Autodesk Inventor part; units mm, degrees
ref_plane "YZ Plane" through (0, 0, 0) normal (1, 0, 0) x (0, 1, 0)
ref_plane "XZ Plane" through (0, 0, 0) normal (0, 1, 0) x (-1, 0, 0)
ref_plane "XY Plane" through (0, 0, 0) normal (0, 0, 1) x (1, 0, 0)
sketch "Sketch1" plane through (0, 0, 0) normal (0, 1, 0) x (-1, 0, 0)
  line L0 (0, 0) -> (0, -54.7595)
  line L1 (0, -54.7595) -> (17.2816, -61.6681)
  line L2 (0, -54.7595) -> (18.6114, -54.7595) construction
  line L3 (0, -54.7595) -> (28.8848, -66.3067)
  line L4 (28.8848, -66.3067) -> (28.8848, -54.7595)
  line L5 (28.8848, -54.7595) -> (28.8848, 0)
  line L6 (28.8848, 0) -> (28.8848, 11.5473)
  line L7 (28.8848, 11.5473) -> (0, 0)
  line L8 (0, -50.5358) -> (-4, -50.5358)
  line L9 (3.9418, -56.3353) -> (2.457, -60.0495)
  line L10 (2.457, -60.0495) -> (-4, -57.4682)
  line L11 (-4, -57.4682) -> (-4, -50.5358)
  line L12 (28.8848, -66.3067) -> (27.4, -70.0209)
  line L13 (27.4, -70.0209) -> (2.457, -60.0495)
  line L14 (0, -3.5872) -> (-4, -3.5872)
  line L15 (-4, -3.5872) -> (-4, -50.5358)
  line L16 (2.457, 0.9822) -> (0.9721, 4.6964)
  line L17 (0.9721, 4.6964) -> (-4, 2.7087)
  line L18 (-4, 2.7087) -> (-4, -3.5872)
  line L19 (23.3647, 9.3405) -> (21.8799, 13.0547)
  line L20 (21.8799, 13.0547) -> (0.9721, 4.6964)
  line L21 (28.8848, 11.5473) -> (27.4, 15.2615)
  line L22 (27.4, 15.2615) -> (21.8799, 13.0547)
  dimension "d0" = 54.7595
  dimension "d1" = 21.79
  dimension "d2" = 31.1075
  dimension "d3" = 11.5473
  dimension "d4" = 11.5473
  dimension "d5" = 4
  dimension "d6" = 4
  dimension "d7" = 4
extrude "Extrusion1" add sketch "Sketch1" along normal blind 40 contours L0 L14 L18 L17 L16 L7 | L0 L8 L15 L14 | L16 L20 L19 L7 | L0 L1 L9 L10 L11 L8 | L19 L22 L21 L7 | L1 L3 L12 L13 L9
sketch "Sketch2" plane through (0, 0, 0) normal (0, -1, 0) x (1, 0, 0)
  line L0 (0, -54.7595) -> (0, 0)
  line L1 (0, -27.3797) -> (8, -27.3797)
  circle A0 centre (8, -27.3797) radius 1.75
  circle A1 centre (8, -27.3797) radius 3.5
  line L2 (4, 2.7087) -> (4, -57.4682)
  line L3 (4, -27.3797) -> (4, -30.8797)
  line L4 (4, -30.8797) -> (8, -30.8797)
  line L5 (4, -27.3797) -> (4, -23.8797)
  line L6 (4, -23.8797) -> (8, -23.8797)
  line L7 (-27.4, -70.0209) -> (-28.8848, -66.3067)
  line L8 (-28.8848, -66.3067) -> (-27.0288, -70.9495)
  line L9 (-27.0288, -70.9495) -> (-28.8848, -66.3067)
  line L10 (-28.8848, -66.3067) -> (-24.2421, -64.4507)
  line L11 (-24.2421, -64.4507) -> (-21.2724, -71.8791)
  circle A2 centre (-21.2724, -71.8791) radius 1.75
  circle A3 centre (-21.2724, -71.8791) radius 3.5
  line L12 (4, -57.4682) -> (-27.4, -70.0209)
  line L13 (-22.7573, -68.1649) -> (-26.0072, -69.4641)
  line L14 (-26.0072, -69.4641) -> (-24.5224, -73.1783)
  line L15 (-22.7573, -68.1649) -> (-19.5073, -66.8657)
  line L16 (-19.5073, -66.8657) -> (-18.0225, -70.5799)
  line L17 (-28.8848, 11.5473) -> (-24.2421, 9.6912)
  line L18 (0, 0) -> (-28.8848, 11.5473)
  line L19 (-24.2421, 9.6912) -> (-21.2724, 17.1196)
  circle A4 centre (-21.2724, 17.1196) radius 1.75
  circle A5 centre (-21.2724, 17.1196) radius 3.5
  line L20 (-27.4, 15.2615) -> (4, 2.7087)
  line L21 (-22.7573, 13.4054) -> (-26.0072, 14.7047)
  line L22 (-26.0072, 14.7047) -> (-24.5224, 18.4189)
  line L23 (-22.7573, 13.4054) -> (-19.5073, 12.1062)
  line L24 (-19.5073, 12.1062) -> (-18.0225, 15.8204)
  dimension "d10" = 8
  dimension "d11" = 3.5
  dimension "d12" = 7
  dimension "d13" = 5
  dimension "d14" = 5
  dimension "d15" = 8
  dimension "d16" = 3.5
  dimension "d17" = 7
  dimension "d18" = 3.5
  dimension "d19" = 3.5
  dimension "d20" = 5
  dimension "d21" = 3.5
  dimension "d22" = 7
  dimension "d23" = 3.5
extrude "Extrusion2" add sketch "Sketch2" against normal blind 3 contours L16 A3 L11 L12 | L2 L6 A1 L1 | L1 A1 L4 L2 | A1 | L20 L22 A5 L19 | L19 A5 L24 L20 | A5 | L11 A3 L14 L12 | A3
sketch "Sketch3" plane through (0, 40, 0) normal (0, 1, 0) x (1, 0, 0)
  line L0 (4, 23.8797) -> (4, 30.8797)
  line L1 (4, 27.3797) -> (4, 30.8797)
  line L2 (8, 30.8797) -> (4, 30.8797)
  line L3 (4, 30.8797) -> (8, 30.8797)
  line L4 (4, 27.3797) -> (4, 23.8797)
  line L5 (4, 23.8797) -> (8, 23.8797)
  line L6 (4, 23.8797) -> (8, 23.8797)
  circle A0 centre (8, 27.3797) radius 1.75
  circle A1 centre (8, 27.3797) radius 1.75
  circle A2 centre (8, 27.3797) radius 3.5
  point P0 (0, 0)
extrude "Extrusion3" add sketch "Sketch3" against normal blind 3 contours A2
sketch "Sketch4" plane through (0, 40, 0) normal (0, 1, 0) x (1, 0, 0)
  line L0 (4, 23.8797) -> (4, 30.8797)
  line L1 (4, 23.8797) -> (8, 23.8797)
  circle A0 centre (8, 27.3797) radius 3.5
  line L2 (8, 30.8797) -> (4, 30.8797)
  line L3 (4, 30.8797) -> (8, 30.8797)
  point P0 (0, 0)
extrude "Extrusion4" add sketch "Sketch4" against normal blind 3 contours L0 L2 A0 L1
sketch "Sketch5" plane through (0, 40, 0) normal (0, 1, 0) x (1, 0, 0)
  point P0 (0, 0)
fillet "Fillet1" radius 20 4 edges at (0, 20, 0) (0, 20, -54.7595) (4, 20, 2.7087) (4, 20, -57.4682)
properties part number "Capture Zone4"
Build history of the part. All positions in model axes, mm. A direction names the side the tool comes from. Give positions to 0.01 mm unless a question says otherwise; leave off trailing zeros. Loops run counter-clockwise (first coordinate to the right, second up) from the corner with the lowest first, then second, coordinate; pieces in that order, holes last. Notation, with made-up numbers: (77.25, 20.5) - (108.25, 20.5) arc R11 cw to (108.25, 25.5) - close; hole circle Ø9 at (-15.5, 27.5). An arc over 180 degrees is marked (long way). Write item = value, one per line. Start each with the question number.
1) Probe probe 1 along Z at (x, y) = (-3.5, 29.5); probe 2 along X at (y, z) = (26.5, -36.5); probe 3 along Z at (x, y) = (-14, 34.5). List the from-to ranges inside material, lowest first. Write a range as from..to.
2) Band-saw the part on C-C on x = -9.5. Give the cut face in (y, z), plus the area to 3 significant figures.
3) Band-saw the part on B-B on z = -37.5. Give the cut face in (x, y), plus the area to 3 significant figures.
4) Drop flat-ended pins along their axis: pin 1 Ø6 at (y, z) = (13.5, -50) entering from +X; pin 2 Ø10 at (y, z) = (21.5, -34) entering from +X; pin 3 Ø1.5 at (x, y) = (7, 38) entering from +Z. Give the stop position or say it passes through.
5) Tool access for faces 1 (the flat face through (6, 39, -23.88)), 2 (the flat face through (0, 20, -27)), 3 (the flat face through (-22, 3, -70)), 4 (the flat face through (-18.775, 1.479, 13.937)): list every direction of +Z, -Z, +X, -X, +Y, -Y with a clear straight run to the whole face (end or side of a thin tool).
6) Pull direction Z, two halves, no side cores. Call faces 5 (the flat face through (6, 1, -30.88)), 6 (the flat face through (-22, 3, 15)), 7 (the flat face through (-18.775, 1.479, -68.697)): +Z half, -Z half, draft (parallel to the pull), parting line (faces both ways), or undercut.
7) Band-saw the part on A-A on x = -15.5. Give the cut face in (y, z).
Final values:
q1.probe_1 = -59.54..-52.52, -2.24..4.78
q1.probe_2 = 0..4
q1.probe_3 = -64.66..-60.36, 5.6..9.9
q2.outline = (0, -62.87) - (40, -62.87) - (40, -58.24) - (0, -58.24) - close; (0, 3.48) - (40, 3.48) - (40, 8.11) - (0, 8.11) - close
q2.area = 370 mm²
q3.outline = (0, 0) - (4, 0) - (4, 40) - (0, 40) - close
q3.area = 160 mm²
q4.pin_1 = 3.76
q4.pin_2 = 4
q4.pin_3 = -23.88
q5.face_1 = +Z, +X, +Y, -Y
q5.face_2 = -X, +Y, -Y
q5.face_3 = -Z, +X, +Y
q5.face_4 = +X, +Y, -Y
q6.face_5 = -Z half
q6.face_6 = draft
q6.face_7 = undercut
q7.outline = (0, -65.26) - (40, -65.26) - (40, -60.96) - (0, -60.96) - close; (0, 6.2) - (40, 6.2) - (40, 10.5) - (0, 10.5) - close
